from build123d import *

# Parameters (mm, degrees)
F1_DEPTH = 4
F2_R     = 2.5
F3_DEPTH = 1.5
F4_R     = 2.5
F5_DEPTH = 1.5
F6_R     = 2
F7_DEPTH = 25


with BuildPart() as f1:
    # F0 (on Top) → F1 (new body)
    with BuildSketch(Plane.XY):
        Polygon((4.71808, -0.549743), (4.75, 0), (4.71808, 0.549743), (5.165056, 0.601824), (5.611973, 0.654414), (6.042571, 0.835065), (6.451897, 1.12939), (6.835156, 1.510179), (6.761481, 1.811733), (6.674508, 2.109724), (6.152202, 2.247869), (5.650552, 2.298099), (5.187318, 2.239248), (4.773982, 2.061333), (4.360849, 1.882949), (4.113621, 2.375), (3.811106, 2.835132), (4.172158, 3.103723), (4.532904, 3.372726), (4.815488, 3.744473), (5.022812, 4.204029), (5.164329, 4.725432), (4.949747, 4.949747), (4.725432, 5.164329), (4.204029, 5.022812), (3.744473, 4.815488), (3.372726, 4.532904), (3.103723, 4.172158), (2.835132, 3.811106), (2.375, 4.113621), (1.882949, 4.360849), (2.061333, 4.773982), (2.239248, 5.187318), (2.298099, 5.650552), (2.247869, 6.152202), (2.109724, 6.674508), (1.811733, 6.761481), (1.510179, 6.835156), (1.12939, 6.451897), (0.835065, 6.042571), (0.654414, 5.611973), (0.601824, 5.165056), (0.549743, 4.71808), (0, 4.75), (-0.549743, 4.71808), (-0.601824, 5.165056), (-0.654414, 5.611973), (-0.835065, 6.042571), (-1.12939, 6.451897), (-1.510179, 6.835156), (-1.811733, 6.761481), (-2.109724, 6.674508), (-2.247869, 6.152202), (-2.298099, 5.650552), (-2.239248, 5.187318), (-2.061333, 4.773982), (-1.882949, 4.360849), (-2.375, 4.113621), (-2.835132, 3.811106), (-3.103723, 4.172158), (-3.372726, 4.532904), (-3.744473, 4.815488), (-4.204029, 5.022812), (-4.725432, 5.164329), (-4.949747, 4.949747), (-5.164329, 4.725432), (-5.022812, 4.204029), (-4.815488, 3.744473), (-4.532904, 3.372726), (-4.172158, 3.103723), (-3.811106, 2.835132), (-4.113621, 2.375), (-4.360849, 1.882949), (-4.773982, 2.061333), (-5.187318, 2.239248), (-5.650552, 2.298099), (-6.152202, 2.247869), (-6.674508, 2.109724), (-6.761481, 1.811733), (-6.835156, 1.510179), (-6.451897, 1.12939), (-6.042571, 0.835065), (-5.611973, 0.654414), (-5.165056, 0.601824), (-4.71808, 0.549743), (-4.75, 0), (-4.71808, -0.549743), (-5.165056, -0.601824), (-5.611973, -0.654414), (-6.042571, -0.835065), (-6.451897, -1.12939), (-6.835156, -1.510179), (-6.761481, -1.811733), (-6.674508, -2.109724), (-6.152202, -2.247869), (-5.650552, -2.298099), (-5.187318, -2.239248), (-4.773982, -2.061333), (-4.360849, -1.882949), (-4.113621, -2.375), (-3.811106, -2.835132), (-4.172158, -3.103723), (-4.532904, -3.372726), (-4.815488, -3.744473), (-5.022812, -4.204029), (-5.164329, -4.725432), (-4.949747, -4.949747), (-4.725432, -5.164329), (-4.204029, -5.022812), (-3.744473, -4.815488), (-3.372726, -4.532904), (-3.103723, -4.172158), (-2.835132, -3.811106), (-2.375, -4.113621), (-1.882949, -4.360849), (-2.061333, -4.773982), (-2.239248, -5.187318), (-2.298099, -5.650552), (-2.247869, -6.152202), (-2.109724, -6.674508), (-1.811733, -6.761481), (-1.510179, -6.835156), (-1.12939, -6.451897), (-0.835065, -6.042571), (-0.654414, -5.611973), (-0.601824, -5.165056), (-0.549743, -4.71808), (0, -4.75), (0.549743, -4.71808), (0.601824, -5.165056), (0.654414, -5.611973), (0.835065, -6.042571), (1.12939, -6.451897), (1.510179, -6.835156), (1.811733, -6.761481), (2.109724, -6.674508), (2.247869, -6.152202), (2.298099, -5.650552), (2.239248, -5.187318), (2.061333, -4.773982), (1.882949, -4.360849), (2.375, -4.113621), (2.835132, -3.811106), (3.103723, -4.172158), (3.372726, -4.532904), (3.744473, -4.815488), (4.204029, -5.022812), (4.725432, -5.164329), (4.949747, -4.949747), (5.164329, -4.725432), (5.022812, -4.204029), (4.815488, -3.744473), (4.532904, -3.372726), (4.172158, -3.103723), (3.811106, -2.835132), (4.113621, -2.375), (4.360849, -1.882949), (4.773982, -2.061333), (5.187318, -2.239248), (5.650552, -2.298099), (6.152202, -2.247869), (6.674508, -2.109724), (6.761481, -1.811733), (6.835156, -1.510179), (6.451897, -1.12939), (6.042571, -0.835065), (5.611973, -0.654414), (5.165056, -0.601824), align=None)
    extrude(amount=F1_DEPTH)

    # F2 (on face) → F3 (cut)
    with BuildSketch(Plane(origin=(0, 0, 0), x_dir=(1, 0, 0), z_dir=(0, 0, -1))):
        Circle(F2_R)
    extrude(amount=-F3_DEPTH, mode=Mode.SUBTRACT)

    # F4 (on face) → F5 (cut)
    with BuildSketch(Plane.XY.offset(4)):
        Circle(F4_R)
    extrude(amount=-F5_DEPTH, mode=Mode.SUBTRACT)

    # F6 (on face) → F7 (cut)
    with BuildSketch(Plane.XY.offset(2.5)):
        Circle(F6_R)
    extrude(amount=-F7_DEPTH, mode=Mode.SUBTRACT)


solid = f1.part
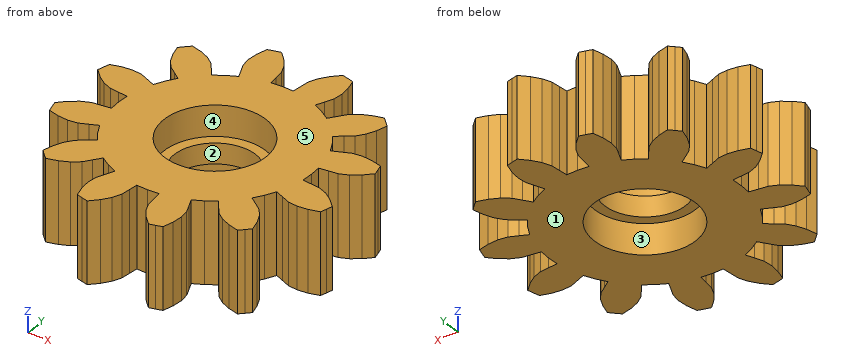
Build history of the part. All positions in model axes, mm. Face numbers are marked on the shaded views. A direction names the side the tool comes from. Coordinates: 2 decimals unless noted, no trailing zeros.
(1) Drill centre lines: line 1 (Y direction, x = 0, z = 3.35); line 2 (Y direction, x = 0, z = 1.8). Where is each one in solid material? Low to high.
(2) 3-axis set-ups, long thin cutter, end or side, ignore diameter. For the marked faces 3, 4 and 5: which of +Z, -Z, +X, -X, +Y, -Y reach the whole face in a straight line?
(3) Mould opens along Y. For the marked faces 1 and 2 say: pulls with the +Y half, pulls with the -Y half, needs draft (parallel to the pull), parting line crosses it, or undercut.
(4) Pin check, flat tips, straight feed: pin 1 Ø5 at (x, y) = (-2, -2.5) entering from -Z; pin 2 Ø4.5 at (x, y) = (0, 0) entering from +Z; pin 3 Ø2 at (y, z) = (-5, 0.5) entering from +X. Stop position of each tip, or through.
Working result:
1. line 1: y = -4.75 to -2.5, 2.5 to 4.75
1. line 2: y = -4.75 to -2, 2 to 4.75
2. face 3: -Z
2. face 4: +Z
2. face 5: +Z, +X, -X, +Y, -Y
3. face 1: needs draft
3. face 2: undercut
4. pin 1: stops at z = 0
4. pin 2: stops at z = 2.5
4. pin 3: stops at x = 5.16
